Read the model definition and answer for the solid it produces. Units are mm, in the model's axes. A direction names the side the tool comes from. Round coordinates to 2 decimals unless told otherwise and drop trailing zeros. Loops run counter-clockwise (first coordinate to the right, second up) from the corner with the lowest first, then second, coordinate; pieces in that order, holes last. Notation, with made-up numbers: (-32, -10) -> (-11, -10) arc R30 cw to (-11, 17) -> close; hole circle Ø5 at (61.25, 22.25). An arc over 180 degrees is marked (long way). Put each result on its own line as item: value.
from build123d import *

# Parameters (mm, degrees)
BOSS_EXTRUDE1_DEPTH = 5
BOSS_EXTRUDE2_DEPTH = 15
BOSS_EXTRUDE3_DEPTH = 15
SKETCH4_R           = 1.8
CUT_EXTRUDE1_DEPTH  = 6
SKETCH6_W           = 14.9
SKETCH6_H           = 20
BOSS_EXTRUDE4_DEPTH = 5
SKETCH8_R           = 1.5
CUT_EXTRUDE3_DEPTH  = 21
SKETCH9_W           = 5
SKETCH9_H           = 55
BOSS_EXTRUDE5_DEPTH = 5
BOSS_EXTRUDE6_DEPTH = 5


with BuildPart() as part:
    # Sketch1 → Boss-Extrude1 (new body)
    with BuildSketch(Plane.XY):
        Polygon((7.370119522, -25.806772908), (27.470119522, -25.806772908), (27.470119522, -10.806772908), (7.470119522, -10.806772908), (7.470119522, 9.193227092), (-7.529880478, 9.193227092), (-7.529880478, -25.806772908), align=None)
    extrude(amount=BOSS_EXTRUDE1_DEPTH)

    # Sketch4 → Cut-Extrude1 (cut, through all)
    with BuildSketch(Plane(origin=(0, 0, 0), x_dir=(-1, 0, 0), z_dir=(0, 0, -1))):
        with Locations((0.029880478, 1.693227092)):
            Circle(SKETCH4_R)
        with Locations((-19.970119522, -18.306772908)):
            Circle(SKETCH4_R)
    extrude(amount=-CUT_EXTRUDE1_DEPTH, mode=Mode.SUBTRACT)

    # Sketch6 → Boss-Extrude4 (add)
    with BuildSketch(Plane.XY.offset(5)):
        with Locations((-0.079880478, -35.806772908)):
            Rectangle(SKETCH6_W, SKETCH6_H)
    extrude(amount=-BOSS_EXTRUDE4_DEPTH)

    # Sketch8 → Cut-Extrude3 (cut, through all)
    with BuildSketch(Plane.XY.offset(5)):
        with Locations((0, -35.806772908)):
            Circle(SKETCH8_R)
    extrude(amount=-CUT_EXTRUDE3_DEPTH, mode=Mode.SUBTRACT)



with BuildPart() as body_2:
    # Sketch2 → Boss-Extrude2 (new body)
    with BuildSketch(Plane(origin=(0, 0, 0), x_dir=(-1, 0, 0), z_dir=(0, 0, -1))):
        Polygon((-7.470119522, 9.193227092), (-12.470119522, 9.193227092), (-12.470119522, -5.806772908), (-27.470119522, -5.806772908), (-27.470119522, -10.806772908), (-7.470119522, -10.806772908), align=None)
    extrude(amount=BOSS_EXTRUDE2_DEPTH)


with BuildPart() as body_3:
    # Sketch3 → Boss-Extrude3 (new body)
    with BuildSketch(Plane(origin=(0, 0, 0), x_dir=(-1, 0, 0), z_dir=(0, 0, -1))):
        Polygon((7.529880478, 9.193227092), (12.529880478, 9.193227092), (12.529880478, -45.806772908), (7.529880478, -45.806772908), (7.529880478, -25.806772908), align=None)
    extrude(amount=BOSS_EXTRUDE3_DEPTH)


with BuildPart() as part_1:
    add(part.part)

    add(body_3.part)  # Boss-Extrude5 merges body 3
    # Sketch9 → Boss-Extrude5 (add)
    with BuildSketch(Plane.XY.offset(5)):
        with Locations((-10.029880478, -18.306772908)):
            Rectangle(SKETCH9_W, SKETCH9_H)
    extrude(amount=-BOSS_EXTRUDE5_DEPTH)


    add(body_2.part)  # Boss-Extrude6 merges body 2
    # Sketch10 → Boss-Extrude6 (add)
    with BuildSketch(Plane.XY):
        Polygon((7.470119522, 9.193227092), (12.470119522, 9.193227092), (12.470119522, -5.806772908), (27.470119522, -5.806772908), (27.470119522, -10.806772908), (7.470119522, -10.806772908), align=None)
    extrude(amount=BOSS_EXTRUDE6_DEPTH)


solid = part_1.part
Item 1: The part is cut by section D-D (x = 0). Determine the outline of the cut face in (y, z).
Derived:
outline: (-45.81, 0) -> (-37.31, 0) -> (-37.31, 5) -> (-45.81, 5) -> close; (-34.31, 0) -> (-0.11, 0) -> (-0.11, 5) -> (-34.31, 5) -> close; (3.49, 0) -> (9.19, 0) -> (9.19, 5) -> (3.49, 5) -> close
Item 2: Which of the six approach directions +Z, -Z, +X, -X, +Y, -Y give full straight-line access (tool end or side, diameter ignored) to faces 1 (the flat face through (7.37, -36, 3)), 2 (the flat face through (18, -10.807, -7)), 3 (the flat face through (7.47, -1, -7))?
Derived:
face 1: +Z, -Z, +X, -Y
face 2: -Z, +X, -Y
face 3: -Z, +Y, -Y
Item 3: The part is cut by section B-B (y = -31.5). Determine the outline of the cut face in (x, z), then the cut area to 4 significant figures.
Derived:
outline: (-12.53, -15) -> (-7.53, -15) -> (-7.53, 0) -> (7.37, 0) -> (7.37, 5) -> (-12.53, 5) -> close
area: 174.5 mm^2
Item 4: For a pull along X with two mould halves and no side action, classify faces 4 (the flat face through (-12.53, -19, -5)), 5 (the flat face through (27.47, -11, 2)), 6 (the flat face through (20, -5.807, -5)), 7 (the flat face through (-7.53, -18, -7)) as pulls with the +X half, pulls with the -X half, needs draft (parallel to the pull), parting line crosses it, or undercut.
Derived:
face 4: pulls with the -X half
face 5: pulls with the +X half
face 6: needs draft
face 7: undercut
Item 5: The part is cut by section C-C (x = 15). Determine the outline of the cut face in (y, z).
Derived:
outline: (-25.81, 0) -> (-10.81, 0) -> (-10.81, -15) -> (-5.81, -15) -> (-5.81, 5) -> (-25.81, 5) -> close
Item 6: Flat-ended cylindrical pins translate along their axes: pin 1 Ø10 at (x, z) = (-7, -12.5) entering from +Y; pin 2 Ø7.5 at (y, z) = (-25, -4.5) entering from +X; pin 3 Ø4.5 at (x, z) = (21.5, -7.5) entering from -Y; pin 4 Ø4.5 at (y, z) = (-1, -6.5) entering from +X. Find the tip coordinate at first contact, or state that the pin passes through.
Derived:
pin 1: stops at y = 9.19
pin 2: stops at x = -7.53
pin 3: stops at y = -10.81
pin 4: stops at x = 12.47
Item 7: The part is cut by section A-A (z = -3.75). Determine the outline of the cut face in (x, y), then the cut area to 3 significant figures.
Derived:
outline: (-12.53, -45.81) -> (-7.53, -45.81) -> (-7.53, 9.19) -> (-12.53, 9.19) -> close; (7.47, -10.81) -> (27.47, -10.81) -> (27.47, -5.81) -> (12.47, -5.81) -> (12.47, 9.19) -> (7.47, 9.19) -> close
area: 450 mm^2
Item 8: Find the intervals of material crossed by line 1 along Y through (x, z) = (0, 1.8); line 2 along X through (y, z) = (1.5, -11.25); line 3 along Z through (x, y) = (2.5, 3.5), in increasing order.
Derived:
line 1: y = -45.81 to -37.31, -34.31 to -0.11, 3.49 to 9.19
line 2: x = -12.53 to -7.53, 7.47 to 12.47
line 3: z = 0 to 5
